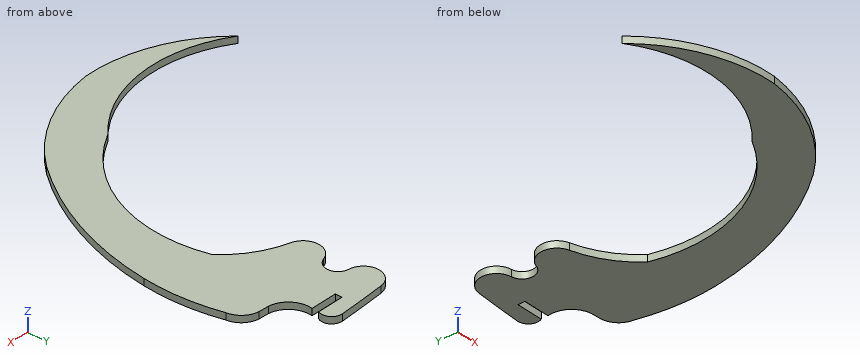
from build123d import *

# Parameters (mm, degrees)
BOSS_EXTRUDE1_DEPTH = 1.524


with BuildPart() as part:
    # Sketch1 → Boss-Extrude1 (new body)
    with BuildSketch(Plane.XY):
        with BuildLine():
            Line((8.098483712, 11.859727981), (5.877367718, 11.949858026))
            ThreePointArc((5.877367718, 11.949858026), (2.370350057, 13.962618774), (1.378838723, 17.882731524))
            Line((1.378838723, 17.882731524), (-4.494535751, 17.881911563))
            Line((-4.494535751, 17.881911563), (-4.494535751, 19.408886177))
            Line((-4.494535751, 19.408886177), (1.380889641, 19.408886177))
            ThreePointArc((1.380889641, 19.408886177), (1.19021021, 21.756216477), (-0.921759528, 22.798282696))
            ThreePointArc((-0.921759528, 22.798282696), (-6.208886665, 22.451672785), (-11.489936734, 22.022298875))
            ThreePointArc((-11.489936734, 22.022298875), (-14.876191758, 18.331465892), (-11.509843158, 14.622467604))
            ThreePointArc((-11.509843158, 14.622467604), (-9.080668933, 12.21547028), (-10.965433597, 9.362018739))
            ThreePointArc((-10.965433597, 9.362018739), (-13.682519769, 5.593287076), (-10.802877432, 1.947254215))
            ThreePointArc((-10.802877432, 1.947254215), (-4.434214721, -0.855352195), (0.739102642, -5.50844309))
            ThreePointArc((0.739102642, -5.50844309), (-0.02520916, -26.956652298), (-14.27594324, -43.004282308))
            ThreePointArc((-14.27594324, -43.004282308), (-31.998801932, -51.188810857), (-50.921597015, -46.391514323))
            ThreePointArc((-50.921597015, -46.391514323), (-38.979769068, -54.843194408), (-24.585605901, -57.4597222))
            ThreePointArc((-24.585605901, -57.4597222), (-11.010595968, -53.177928069), (0, -44.156762285))
            ThreePointArc((0, -44.156762285), (9.481977012, -27.77313527), (13.853593601, -9.35520676))
            ThreePointArc((13.853593601, -9.35520676), (13.803097482, -0.628370713), (12.139120175, 7.938507176))
            ThreePointArc((12.139120175, 7.938507176), (10.799936026, 10.60099471), (8.098483712, 11.859727981))
        make_face()
    extrude(amount=BOSS_EXTRUDE1_DEPTH)


solid = part.part
The model under review builds one solid part; all positions refer to its coordinate system, in mm. Coordinates: 2 decimals unless noted, no trailing zeros. Write each loop counter-clockwise with the first axis right and the second up, starting at its lowest first coordinate (ties: lowest second). Pieces come first, ordered by that corner, then holes. Notation, with made-up numbers: M 87.25,-27.75 L 132.25,-27.75 A17 cw 132.25,-23.75 Z; hole C 75.5,29.25 d8. An arc over 180 degrees is marked long. Put each result on its own line as item: value.
1) Clearance check with a flat-ended pin moving along its axis: pin 1 Ø0.8 at (y, z) = (18.5, 1) entering from +X. State where the tip first meets the part, or that it passes through.
Computed:
pin 1: stops at x = -4.49
2) Add section A-A on z = 0.7. Give the boundary of the cut face in (x, y).
Computed:
outline: M -50.92,-46.39 A33.82 ccw -24.59,-57.46 A37.6 ccw 0,-44.16 A65.15 ccw 13.85,-9.36 A46.97 ccw 12.14,7.94 A4.54 ccw 8.1,11.86 L 5.88,11.95 A5.18 cw 1.38,17.88 L -4.49,17.88 L -4.49,19.41 L 1.38,19.41 A2.39 ccw -0.92,22.8 A338.29 ccw -11.49,22.02 A3.72 ccw -11.51,14.62 A2.7 cw -10.97,9.36 A3.86 ccw -10.8,1.95 A21.98 cw 0.74,-5.51 A31.71 cw -14.28,-43 A29.23 cw Z
3) Add section B-B on x = -17.5. Give the boundary of the cut face in (y, z), then the cut area to 3 significant figures.
Computed:
outline: M -55.94,0 L -45.72,0 L -45.72,1.52 L -55.94,1.52 Z
area: 15.6 mm2
4) Wall thickness on probe 1 along Y at (x, z) = (-2, 1.4); probe 2 along Y at (x, z) = (-3.5, 0.5); probe 3 along X at (y, z) = (-8.5, 0.25): over which ranges is each line inside the solid? List them lowest first. Write a range as [from, to].
Computed:
probe 1: y = [-46.38, -31.02], [-2.68, 17.88], [19.41, 22.73]
probe 2: y = [-47.83, -33.37], [-1.49, 17.88], [19.41, 22.64]
probe 3: x = [1.54, 13.92]
5) Add section C-C on y = -45. Give the boundary of the cut face in (x, z), then the cut area to 3 significant figures.
Computed:
outline: M -16.55,0 L -0.72,0 L -0.72,1.52 L -16.55,1.52 Z
area: 24.1 mm2
